For this review, take the finished solid that the model builds, in its own axes (mm). Face numbers are marked on the shaded views. Round coordinates to 2 decimals unless told otherwise and drop trailing zeros. Order: outer loops, then holes, each group sorted by start corner. A loop starts at its lowest first (then second) coordinate and runs counter-clockwise, first axis right, second up. Notation, with made-up numbers: (7.5, 15.25) -> (19.5, 15.25) arc R21 cw to (19.5, 50.25) -> close; hole circle Ø8 at (45, 27). An arc over 180 degrees is marked (long way). Use a Markdown table: item, result. Add a question column.
1) Consider section A-A (y = 0). State the section outline as (x, z) points, plus the area to 3 significant figures.
2) Consider section C-C (x = 6.5). State the section outline as (y, z) points, plus the area to 3 significant figures.
3) Wall thickness on line 1 along Y through (x, z) = (2, 6.5); line 2 along Z through (x, y) = (4.25, 2.5); line 3 along Z through (x, y) = (5.75, -3): over which ranges is each line inside the solid? List them lowest first. Write a range as [from, to].
4) Consider section D-D (z = 0). State the section outline as (x, y) points, plus the area to 3 significant figures.
5) Draft analysis for pull direction Z (two halves, no side actions). For the marked faces 1, 2 and 3, state which applies: pulls with the +Z half, pulls with the -Z half, needs draft (parallel to the pull), parting line crosses it, or undercut.
6) Clearance check with a flat-ended pin moving along its axis: P1, Ø1.3, axis at y = 1, z = 1, coming from the +X side. State where the tip first meets the part, or that it passes through.
7) Consider section B-B (z = 6.5). State the section outline as (x, y) points.
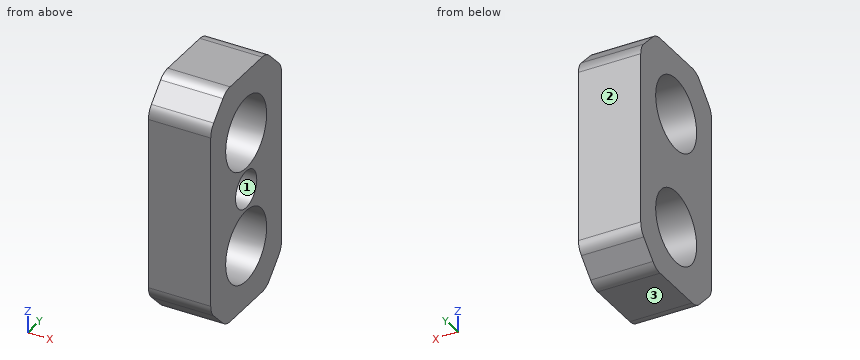
```python
from build123d import *

# Parameters (mm, degrees)
SKETCH1_W           = 27
SKETCH1_H           = 14
SKETCH1_R           = 4.05
BOSS_EXTRUDE1_DEPTH = 7
SKETCH3_R           = 2.1
CUT_EXTRUDE4_DEPTH  = 5
CHANFREIN1_SIZE     = 3
CONG_1_R            = 2


with BuildPart() as part:
    # Sketch1 → Boss-Extrude1 (new body)
    with BuildSketch(Plane(origin=(0, 0, 0), x_dir=(0, 0, -1), z_dir=(1, 0, 0))):
        Rectangle(SKETCH1_W, SKETCH1_H)
        with Locations((-6.5, 0)):
            Circle(SKETCH1_R, mode=Mode.SUBTRACT)
        with Locations((6.5, 0)):
            Circle(SKETCH1_R, mode=Mode.SUBTRACT)
    extrude(amount=BOSS_EXTRUDE1_DEPTH)

    # Sketch3 → Cut-Extrude4 (cut)
    with BuildSketch(Plane(origin=(7, 0, 0), x_dir=(0, 0, -1), z_dir=(1, 0, 0))):
        Circle(SKETCH3_R)
    extrude(amount=-CUT_EXTRUDE4_DEPTH, mode=Mode.SUBTRACT)

    # Chanfrein1
    chanfrein1_edges = [part.edges().sort_by_distance(p)[0] for p in [
        (3.5, 7, 13.5),
        (3.5, 7, -13.5),
        (3.5, -7, -13.5),
        (3.5, -7, 13.5),
    ]]
    chamfer(chanfrein1_edges, length=CHANFREIN1_SIZE)

    # Congé1
    cong_1_edges = [part.edges().sort_by_distance(p)[0] for p in [
        (3.5, -4, 13.5),
        (3.5, 4, 13.5),
        (3.5, 7, -10.5),
        (3.5, 7, 10.5),
        (3.5, -7, -10.5),
        (3.5, -7, 10.5),
        (3.5, 4, -13.5),
        (3.5, -4, -13.5),
    ]]
    fillet(cong_1_edges, radius=CONG_1_R)


solid = part.part
```
Results list:
| question | item | result |
|---|---|---|
| 1 | outline | (0, -13.5) -> (7, -13.5) -> (7, -10.55) -> (0, -10.55) -> close; (0, -2.45) -> (7, -2.45) -> (7, -2.1) -> (2, -2.1) -> (2, 2.1) -> (7, 2.1) -> (7, 2.45) -> (0, 2.45) -> close; (0, 10.55) -> (7, 10.55) -> (7, 13.5) -> (0, 13.5) -> close |
| 1 | area | 54.6 mm2 |
| 2 | outline | (-7, -9.67) arc R2 ccw to (-6.41, -11.09) -> (-4.59, -12.91) arc R2 ccw to (-3.17, -13.5) -> (3.17, -13.5) arc R2 ccw to (4.59, -12.91) -> (6.41, -11.09) arc R2 ccw to (7, -9.67) -> (7, 9.67) arc R2 ccw to (6.41, 11.09) -> (4.59, 12.91) arc R2 ccw to (3.17, 13.5) -> (-3.17, 13.5) arc R2 ccw to (-4.59, 12.91) -> (-6.41, 11.09) arc R2 ccw to (-7, 9.67) -> close; hole circle Ø8.1 at (0, -6.5); hole circle Ø8.1 at (0, 6.5); hole circle Ø4.2 at (0, 0) |
| 2 | area | 242 mm2 |
| 3 | line 1 | [-7, -4.05], [4.05, 7] |
| 3 | line 2 | [-13.5, -9.69], [-3.31, 3.31], [9.69, 13.5] |
| 3 | line 3 | [-13.5, -9.22], [-3.78, 3.78], [9.22, 13.5] |
| 4 | outline | (0, -7) -> (7, -7) -> (7, -2.1) -> (2, -2.1) -> (2, 2.1) -> (7, 2.1) -> (7, 7) -> (0, 7) -> close |
| 4 | area | 77.0 mm2 |
| 5 | face 1 | undercut |
| 5 | face 2 | needs draft |
| 5 | face 3 | pulls with the -Z half |
| 6 | P1 | x = 2 |
| 7 | outline | (0, -7) -> (7, -7) -> (7, -4.05) -> (0, -4.05) -> close; (0, 4.05) -> (7, 4.05) -> (7, 7) -> (0, 7) -> close |
